from build123d import *

# Parameters (mm, degrees)
CROQUIS1_W                 = 12
CROQUIS1_H                 = 12
SALIENTE_EXTRUIR1_DEPTH    = 36
VACIADO1_T                 = -1
CORTAR_EXTRUIR1_DEPTH      = 37.986484018
CORTAR_EXTRUIR1_DEPTH_BACK = 3
CROQUIS2_R                 = 3.25
CROQUIS3_W                 = 13.652855543
CROQUIS3_H                 = 1.6
CORTAR_EXTRUIR2_DEPTH      = 9
CROQUIS4_W                 = 10
CROQUIS4_H                 = 1
SALIENTE_EXTRUIR2_DEPTH    = 11


with BuildPart() as part:
    # Croquis1 → Saliente-Extruir1 (new body)
    with BuildSketch(Plane(origin=(0, 0, 0), x_dir=(1, 0, 0), z_dir=(0, 1, 0))):
        Rectangle(CROQUIS1_W, CROQUIS1_H)
    extrude(amount=SALIENTE_EXTRUIR1_DEPTH)

    # Vaciado1
    vaciado1_openings = [part.faces().sort_by_distance(p)[0] for p in [
        (0, 18, 6),
    ]]
    offset(amount=VACIADO1_T, openings=vaciado1_openings, kind=Kind.INTERSECTION)

    # Croquis2 → Cortar-Extruir1 (cut, two sides: drawn at the far end of the back side and taken through both)
    with BuildSketch(Plane(origin=(0, 36, 0), x_dir=(1, 0, 0), z_dir=(0, 1, 0)).offset(-CORTAR_EXTRUIR1_DEPTH_BACK)):
        with Locations(Location((0, 0, 0), (0, 0, 90))):
            Circle(CROQUIS2_R)
    extrude(amount=CORTAR_EXTRUIR1_DEPTH + CORTAR_EXTRUIR1_DEPTH_BACK, mode=Mode.SUBTRACT)

    # Croquis3 → Cortar-Extruir2 (cut)
    with BuildSketch(Plane.XY.offset(6)):
        with Locations((0.0537514, 1.8)):
            Rectangle(CROQUIS3_W, CROQUIS3_H)
    extrude(amount=-CORTAR_EXTRUIR2_DEPTH, mode=Mode.SUBTRACT)

    # Croquis4 → Saliente-Extruir2 (add)
    with BuildSketch(Plane.XY.offset(6)):
        with Locations((0, 3.1)):
            Rectangle(CROQUIS4_W, CROQUIS4_H)
    extrude(amount=-SALIENTE_EXTRUIR2_DEPTH)


solid = part.part
Geometry check sheet. Reference: the model listing, model coordinates, mm. A direction names the side the tool comes from. Round coordinates to 2 decimals unless told otherwise and drop trailing zeros. Loops run counter-clockwise (first coordinate to the right, second up) from the corner with the lowest first, then second, coordinate; pieces in that order, holes last. Notation, with made-up numbers: (5, 23.25) -> (44, 23.25) arc R12 cw to (44, 29.25) -> close; hole circle Ø7 at (-15, -18). An arc over 180 degrees is marked (long way). Answer as a JSON object with one key per item and string values. Group by question number.
Item 1: Thickness scan on line 1 along Y through (x, z) = (-3, -2.5); line 2 along X through (y, z) = (35.8, 0); line 3 along Y through (x, z) = (5.25, 0.5). Record the ranges inside material, lowest first.
Item 2: Cross-section at B-B, the plane x = 0. Record the cut outline in (y, z), plus the area to 3 significant figures.
Item 3: Release check for a two-part mould opening along X. For faces 1 (the face through (2, 35, 3)), 2 (the face through (-6, 18, 0)), 3 (the face through (3, 36, -3)) record: pulls with the +X half, pulls with the -X half, needs draft (parallel to the pull), parting line crosses it, or undercut.
Item 4: Cross-section at C-C, the plane y = 18.5. Record the cut outline in (x, z), plus the area to 3 significant figures.
Item 5: Depth check by flat-ended pin: pin 1 Ø5 at (x, z) = (0, 0) entering from +Y; pin 2 Ø0.5 at (x, y) = (0, 1.5) entering from +Z. Enter the tip coordinate at first touch or a pass-through.
Item 6: Cross-section at A-A, the plane z = 0. Record the cut outline in (x, y).
Item 7: Set-up check for faces 4 (the face through (5, 2, -4)), 5 (the face through (-5.5, 1.8, -3)), 6 (the face through (1.978, 35.493, 2.579)), 7 (the face through (0, 0, 0)): record each of +Z, -Z, +X, -X, +Y, -Y from which the full face is reachable in a straight line by a thin tool's end or side.
Determined:
{
 "1": {"line 1": "y = 0 to 1, 2.6 to 3.6, 35 to 36", "line 2": "x = -6 to -3.25, 3.25 to 6", "line 3": "y = 0 to 1, 2.6 to 36"},
 "2": {"outline": "(0, -6) -> (36, -6) -> (36, -3.25) -> (35, -3.25) -> (35, -5) -> (3.6, -5) -> (3.6, 6) -> (2.6, 6) -> (2.6, -5) -> (1, -5) -> (1, 6) -> (0, 6) -> close; (35, 3.25) -> (36, 3.25) -> (36, 6) -> (35, 6) -> close", "area": "62.5 mm²"},
 "3": {"face 1": "undercut", "face 2": "pulls with the -X half", "face 3": "needs draft"},
 "4": {"outline": "(-6, -6) -> (6, -6) -> (6, 6) -> (5, 6) -> (5, -5) -> (-5, -5) -> (-5, 6) -> (-6, 6) -> close", "area": "34.0 mm²"},
 "5": {"pin 1": "stops at y = 3.6", "pin 2": "stops at z = -5"},
 "6": {"outline": "(-6, 0) -> (6, 0) -> (6, 1) -> (-6, 1) -> close; (-6, 2.6) -> (6, 2.6) -> (6, 36) -> (3.25, 36) -> (3.25, 35) -> (5, 35) -> (5, 3.6) -> (-5, 3.6) -> (-5, 35) -> (-3.25, 35) -> (-3.25, 36) -> (-6, 36) -> close"},
 "7": {"face 4": "+Z", "face 5": "+Z, +X, -X", "face 6": "+Y", "face 7": "+Z, -Z, +X, -X, -Y"}
}
